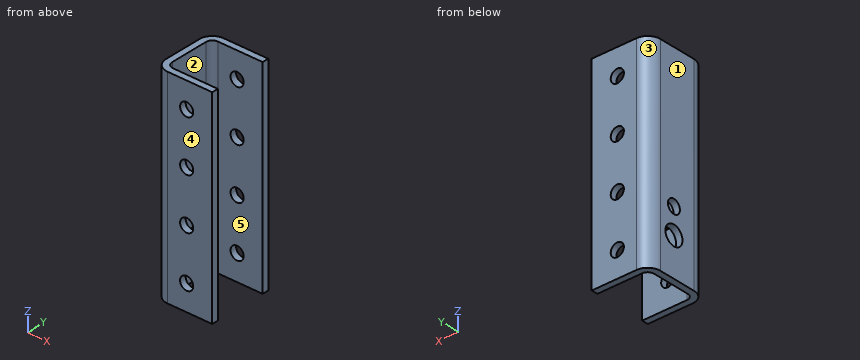
Autodesk Inventor part; units mm, degrees
ref_plane "YZ Plane" through (0, 0, 0) normal (1, 0, 0) x (0, 1, 0)
ref_plane "XZ Plane" through (0, 0, 0) normal (0, 1, 0) x (-1, 0, 0)
ref_plane "XY Plane" through (0, 0, 0) normal (0, 0, 1) x (1, 0, 0)
sketch "Sketch1" plane through (0, 0, 0) normal (0, 0, 1) x (1, 0, 0)
  line L0 (5.9771, 0) -> (28.2021, 0)
  line L1 (28.2021, 0) -> (28.2021, 3.175)
  line L2 (28.2021, 3.175) -> (5.9771, 3.175)
  line L3 (2.8021, 6.35) -> (2.8021, 25.4)
  line L4 (5.9771, 28.575) -> (28.2021, 28.575)
  line L5 (28.2021, 28.575) -> (28.2021, 31.75)
  line L6 (28.2021, 31.75) -> (5.9771, 31.75)
  line L7 (-0.3729, 25.4) -> (-0.3729, 6.35)
  arc A0 (5.9771, 28.575) -> (2.8021, 25.4) centre (5.9771, 25.4) ccw
  arc A1 (2.8021, 6.35) -> (5.9771, 3.175) centre (5.9771, 6.35) ccw
  arc A2 (5.9771, 31.75) -> (-0.3729, 25.4) centre (5.9771, 25.4) ccw
  arc A3 (-0.3729, 6.35) -> (5.9771, 0) centre (5.9771, 6.35) ccw
  point P0 (0, 0)
  point P1 (-0.3729, 0)
  point P2 (2.8021, 3.175)
  point P3 (2.8021, 28.575)
  dimension "d0" = 28.575
  dimension "d1" = 3.175
  dimension "d2" = 25.4
  dimension "d3" = 25.4
  dimension "d4" = 3.175
  dimension "d5" = 3.175
  dimension "d6" = 6.35
extrude "Extrusion1" add sketch "Sketch1" against normal blind 889
sketch "Sketch2" plane through (-0.3729, 6.35, 0) normal (-1, 0, 0) x (0, 0, 1)
  line L0 (0, 19.05) -> (-889, 19.05)
  line L1 (-228.6, 0) -> (-228.6, 7.9375)
  arc A0 (-228.6, 11.1125) -> (-228.6, 7.9375) centre (-228.6, 9.525) ccw
  line L2 (-228.6, 11.1125) -> (-228.6, 19.05)
  line L3 (-228.6, 19.05) -> (-889, 19.05)
  line L4 (-889, 0) -> (-889, 19.05)
  line L5 (-889, 0) -> (-228.6, 0)
  circle A1 centre (-552.45, 11.43) radius 4.826
  circle A2 centre (-501.65, 11.43) radius 4.826
  circle A3 centre (-387.35, 11.43) radius 4.826
  circle A4 centre (-336.55, 11.43) radius 4.826
  circle A5 centre (-444.5, 7.62) radius 4.826
  circle A6 centre (-730.25, 11.43) radius 4.826
  circle A7 centre (-781.05, 11.43) radius 4.826
  line L6 (0, 25.4) -> (-889, 25.4) construction
  circle A8 centre (-133.35, 11.43) radius 4.826
  circle A9 centre (-82.55, 11.43) radius 4.826
  point P0 (0, -6.35)
  point P1 (-254, 0.852)
  dimension "d10" = 7.62
  dimension "d11" = 3.81
  dimension "d14" = 254
hole "Hole1" at (-0.3729, 17.78, -781.05) at (-0.3729, 17.78, -730.25) at (-0.3729, 17.78, -552.45) at (-0.3729, 17.78, -501.65) at (-0.3729, 13.97, -444.5) at (-0.3729, 17.78, -387.35) at (-0.3729, 17.78, -336.55) at (-0.3729, 17.78, -133.35) at (-0.3729, 17.78, -82.55) direction (1, 0, 0) diameter 9.652 end through all
hole "Hole2" at (-0.3729, 15.875, -228.6) direction (1, 0, 0) diameter 3.175 end through all
sketch "Sketch3" plane through (5.9771, 31.75, 0) normal (0, 1, 0) x (1, 0, 0)
  line L0 (22.225, 889) -> (0, 889)
  line L1 (22.225, 0) -> (22.225, 889)
  point P0 (-5.9771, 0)
  point P1 (9.525, 876.3)
  dimension "d34" = 12.7
  dimension "d35" = 12.7
hole "Hole3" at (15.5021, 31.75, -876.3) direction (0, -1, 0) diameter 6.5278 end through all
pattern_linear "Rectangular Pattern1" count 35 spacing 25.4 along (0, 0, 1) of "Hole3"
sketch "Sketch4" plane through (0, 0, -889) normal (0, 0, -1) x (-1, 0, 0)
  line L0 (-28.2021, 0) -> (-28.2021, 3.175)
  line L1 (-5.9771, 0) -> (-28.2021, 0)
  arc A0 (-5.9771, 0) -> (0.3729, 6.35) centre (-5.9771, 6.35) ccw
  line L2 (0.3729, 25.4) -> (0.3729, 6.35)
  arc A1 (0.3729, 25.4) -> (-5.9771, 31.75) centre (-5.9771, 25.4) ccw
  line L3 (-28.2021, 31.75) -> (-5.9771, 31.75)
  line L4 (-28.2021, 28.575) -> (-28.2021, 31.75)
  line L5 (-5.9771, 28.575) -> (-28.2021, 28.575)
  arc A2 (-2.8021, 25.4) -> (-5.9771, 28.575) centre (-5.9771, 25.4) ccw
  line L6 (-2.8021, 6.35) -> (-2.8021, 25.4)
  arc A3 (-5.9771, 3.175) -> (-2.8021, 6.35) centre (-5.9771, 6.35) ccw
  line L7 (-28.2021, 3.175) -> (-5.9771, 3.175)
  point P0 (0, 0)
extrude "Extrusion2" cut sketch "Sketch4" against normal blind 787.4
sketch "Sketch5" plane through (-0.3729, 6.35, 0) normal (-1, 0, 0) x (0, 0, 1)
  line L0 (0, 19.05) -> (-101.6, 19.05)
  circle A0 centre (-82.55, 11.43) radius 4.826
  circle A1 centre (-69.85, 11.43) radius 3.3782
  line L1 (-82.55, 11.43) -> (-69.85, 11.43) construction
  point P0 (0, -6.35)
  dimension "d48" = 6.7564
  dimension "d49" = 12.7
extrude "Extrusion3" cut sketch "Sketch5" against normal blind 25.4 contours A1
properties part number "C Channel Mechanical Stop"
Can you work these out from the model? Positions are in its coordinate system, mm. Face numbers are marked on the shaded views. A direction names the side the tool comes from. Coordinates: 2 decimals unless noted, no trailing zeros. Write each loop counter-clockwise with the first axis right and the second up, starting at its lowest first coordinate (ties: lowest second). Pieces come first, ordered by that corner, then holes.
Q1. Imagine slicing it at A-A, the plane z = -12.7. List the corners of the cut face in (x, y) for me (3 decimals), plus the area to 3 significant figures.
Results found:
outline: (-0.373, 6.35) arc R6.35 ccw to (5.977, 0) - (12.238, 0) - (12.238, 3.175) - (5.977, 3.175) arc R3.175 cw to (2.802, 6.35) - (2.802, 25.4) arc R3.175 cw to (5.977, 28.575) - (12.238, 28.575) - (12.238, 31.75) - (5.977, 31.75) arc R6.35 ccw to (-0.373, 25.4) - close; (18.766, 0) - (28.202, 0) - (28.202, 3.175) - (18.766, 3.175) - close; (18.766, 28.575) - (28.202, 28.575) - (28.202, 31.75) - (18.766, 31.75) - close
area: 208 mm2
Q2. Imagine slicing it at C-C, the plane x = 4. List the corners of the cut face in (y, z) for me.
Results found:
outline: (0.32, -101.6) - (3.87, -101.6) - (3.87, 0) - (0.32, 0) - close; (27.88, -101.6) - (31.43, -101.6) - (31.43, 0) - (27.88, 0) - close
Q3. Which directions (+Z, -Z, +X, -X, +Y, -Y) give clear straight access to the entire face, cutting with the end or side of a thin tool? Please do the marked faces 1 and 2.
Results found:
face 1: +Z, -Z, -X, +Y, -Y
face 2: +Z, -Z, +X
Q4. Imagine slicing it at D-D, the plane z = -69.85. List the corners of the cut face in (x, y) for me (3 decimals), plus the area to 3 significant figures.
Results found:
outline: (-0.373, 6.35) arc R6.35 ccw to (5.977, 0) - (28.202, 0) - (28.202, 3.175) - (5.977, 3.175) arc R3.175 cw to (2.802, 6.35) - (2.802, 14.402) - (-0.373, 14.402) - close; (-0.373, 21.158) - (2.802, 21.158) - (2.802, 25.4) arc R3.175 cw to (5.977, 28.575) - (28.202, 28.575) - (28.202, 31.75) - (5.977, 31.75) arc R6.35 ccw to (-0.373, 25.4) - close
area: 228 mm2
Q5. Imagine slicing it at B-B, the plane y = 17.78. List the corners of the cut face in (x, z) for me.
Results found:
outline: (-0.37, -101.6) - (2.8, -101.6) - (2.8, -87.38) - (-0.37, -87.38) - close; (-0.37, -77.72) - (2.8, -77.72) - (2.8, -73.23) - (-0.37, -73.23) - close; (-0.37, -66.47) - (2.8, -66.47) - (2.8, 0) - (-0.37, 0) - close
Q6. If we mould it in two halves opening along Y, with no side actions, what happens to the marked faces 3, 4 and 5? For each: +Y half, -Y half, draft (parallel to the pull), parting line (faces both ways), or undercut.
Results found:
face 3: +Y half
face 4: -Y half
face 5: undercut
Q7. Please list where these lines run through material, in increasing order: L1, parallel to Y at x = 23, z = -43 (3 decimals); L2, parallel to X at y = 17.5, z = -97; L3, parallel to Y at x = 3.25, z = -56.
Results found:
L1: y = 0 to 3.175, 28.575 to 31.75
L2: x = -0.37 to 2.8
L3: y = 0.62 to 4.72, 27.03 to 31.13
Q8. For P1, Ø9.5, axis at y = 20.5, z = -63, coming from the +X side; P2, Ø4, axis at x = 15.5, z = -88.9, coming from the +Y side, each with a flat end and sliding along its axis, tell me the tip position at first contact or that it passes through.
Results found:
P1: stops at x = 2.8
P2: passes through
